Model file for the job. Use its own axes, mm. A direction names the side the tool comes from. Round coordinates to 2 decimals unless told otherwise and drop trailing zeros. Loops run counter-clockwise (first coordinate to the right, second up) from the corner with the lowest first, then second, coordinate; pieces in that order, holes last. Notation, with made-up numbers: (71, 88.5) -> (102, 88.5) arc R15 cw to (102, 95.5) -> close; hole circle Ø8 at (76, 7.5). An arc over 180 degrees is marked (long way). Use a Markdown table: item, result.
from build123d import *

# Parameters (mm, degrees)
SKETCH_1_R          = 15
EXTRUDE_1_DEPTH     = 80
SKETCH_2_W          = 200
SKETCH_2_H          = 40
CUT_EXTRUDE_1_DEPTH = 125


with BuildPart() as part:
    # 草图1 → 凸台-拉伸1 (new body)
    with BuildSketch(Plane(origin=(0, 0, 0), x_dir=(1, 0, 0), z_dir=(0, 1, 0))):
        with BuildLine():
            Line((-125, 50), (125, 50))
            ThreePointArc((125, 50), (175, 0), (125, -50))
            Line((125, -50), (-125, -50))
            ThreePointArc((-125, -50), (-175, 0), (-125, 50))
        make_face()
        with Locations(Location((-125, 0, 0), (0, 0, 270))):
            Circle(SKETCH_1_R, mode=Mode.SUBTRACT)
        with Locations(Location((125, 0, 0), (0, 0, 270))):
            Circle(SKETCH_1_R, mode=Mode.SUBTRACT)
    extrude(amount=EXTRUDE_1_DEPTH)

    # 草图2 → 切除-拉伸1 (cut)
    with BuildSketch(Plane.XY.offset(50)):
        with Locations((-125, 40)):
            Rectangle(SKETCH_2_W, SKETCH_2_H)
        with Locations((125, 40)):
            Rectangle(SKETCH_2_W, SKETCH_2_H)
    extrude(amount=-CUT_EXTRUDE_1_DEPTH, mode=Mode.SUBTRACT)


solid = part.part
Q1. Band-saw the part on B-B, the plane x = -98. Give the cut face in (y, z), plus the area to 3 significant figures.
Results list:
| item | result |
|---|---|
| outline | (0, -50) -> (20, -50) -> (20, 50) -> (0, 50) -> close; (60, -50) -> (80, -50) -> (80, 50) -> (60, 50) -> close |
| area | 4,000 mm² |
Q2. Band-saw the part on C-C, the plane y = 11. Give the cut face in (x, z).
Results list:
| item | result |
|---|---|
| outline | (-125, -50) -> (125, -50) arc R50 ccw to (125, 50) -> (-125, 50) arc R50 ccw to start; hole circle Ø30 at (-125, 0); hole circle Ø30 at (125, 0) |
Q3. Band-saw the part on A-A, the plane z = 0. Give the cut face in (x, y), plus the area to 3 significant figures.
Results list:
| item | result |
|---|---|
| outline | (-175, 0) -> (-140, 0) -> (-140, 20) -> (-175, 20) -> close; (-175, 60) -> (-140, 60) -> (-140, 80) -> (-175, 80) -> close; (-110, 0) -> (110, 0) -> (110, 20) -> (25, 20) -> (25, 60) -> (110, 60) -> (110, 80) -> (-110, 80) -> (-110, 60) -> (-25, 60) -> (-25, 20) -> (-110, 20) -> close; (140, 0) -> (175, 0) -> (175, 20) -> (140, 20) -> close; (140, 60) -> (175, 60) -> (175, 80) -> (140, 80) -> close |
| area | 13,600 mm² |
Q4. Pull direction X, two halves, no side cores. Call faces 1 (the face through (-174.988, 9.86, 1.099)), 2 (the face through (99, 60, 1)), 3 (the face through (-110.128, 9.86, -1.953)), 4 (the face through (174.988, 69.86, -1.099)): released by +X, released by -X, zero draft, split by the parting line, or undercut.
Results list:
| item | result |
|---|---|
| face 1 | released by -X |
| face 2 | zero draft |
| face 3 | undercut |
| face 4 | released by +X |
Q5. Drill centre lines: L1, parallel to X at y = 73, z = 0; L2, parallel to Y at x = 33.5, z = -17.5; L3, parallel to Z at x = 125, y = 68.5. Where is each one in solid material? Low to high. Write a range as from..to.
Results list:
| item | result |
|---|---|
| L1 | x = -175..-140, -110..110, 140..175 |
| L2 | y = 0..20, 60..80 |
| L3 | z = -50..-15, 15..50 |
Q6. Flat gauge pins, fed straight in: pin 1 (4 mm diameter, centred on y = 23, z = -0.5, fed in from +X); pin 2 (3 mm diameter, centred on y = 10, z = -26.5, fed in from -X); pin 3 (12 mm diameter, centred on y = 58.5, z = 30.5, fed in from +X). Where does each tip first touch, or does it go through?
Results list:
| item | result |
|---|---|
| pin 1 | stops at x = 25 |
| pin 2 | stops at x = -168.3 |
| pin 3 | stops at x = 168.48 |
Q7. Tool access for faces 5 (the face through (-110.128, 69.86, -1.953)), 6 (the face through (-101, 60, 1)), 7 (the face through (99, 20, 1)): list every direction of +Z, -Z, +X, -X, +Y, -Y with a clear straight run to the whole face (end or side of a thin tool).
Results list:
| item | result |
|---|---|
| face 5 | +Y, -Y |
| face 6 | +Z, -Z, -X |
| face 7 | +Z, -Z, +X |
Q8. Band-saw the part on D-D, the plane z = 23. Give the cut face in (x, y).
Results list:
| item | result |
|---|---|
| outline | (-169.4, 0) -> (169.4, 0) -> (169.4, 20) -> (25, 20) -> (25, 60) -> (169.4, 60) -> (169.4, 80) -> (-169.4, 80) -> (-169.4, 60) -> (-25, 60) -> (-25, 20) -> (-169.4, 20) -> close |
